Source: CAD feature listing. Evaluate the final solid. Frame: model axes, mm. Coordinates: 2 decimals unless noted, no trailing zeros. Order: outer loops, then holes, each group sorted by start corner. A loop starts at its lowest first (then second) coordinate and runs counter-clockwise, first axis right, second up.
```python
from build123d import *

# Parameters (mm, degrees)
MODEL_R             = 0.65
MODEL_R_2           = 2.974594
EXTRUDE_1_DEPTH     = 1
CUT_EXTRUDE_1_DEPTH = 0.1


with BuildPart() as part:
    # Model → Бобышка-Вытянуть1 (new body)
    with BuildSketch(Plane.XY):
        with BuildLine():
            Line((-10.4, -5.5), (-4.7, -5.5))
            Line((-4.7, -5.5), (-0.65, -5.5))
            Line((-0.65, -5.5), (-0.65, -4.7))
            ThreePointArc((-0.65, -4.7), (0, -4.05), (0.65, -4.7))
            Line((0.65, -4.7), (0.65, -5.5))
            Line((0.65, -5.5), (3.6, -5.5))
            Line((3.6, -5.5), (5.6, -5.5))
            ThreePointArc((5.6, -5.5), (6.660660172, -5.060660172), (7.1, -4))
            Line((7.1, -4), (7.1, -1.6))
            Line((7.1, -1.6), (7.1, 1.6))
            Line((7.1, 1.6), (7.1, 4))
            ThreePointArc((7.1, 4), (6.660660172, 5.060660172), (5.6, 5.5))
            Line((5.6, 5.5), (3.6, 5.5))
            Line((3.6, 5.5), (0.65, 5.5))
            Line((0.65, 5.5), (0.65, 4.7))
            ThreePointArc((0.65, 4.7), (0, 4.05), (-0.65, 4.7))
            Line((-0.65, 4.7), (-0.65, 5.5))
            Line((-0.65, 5.5), (-4.7, 5.5))
            Line((-4.7, 5.5), (-10.4, 5.5))
            ThreePointArc((-10.4, 5.5), (-11.460660172, 5.060660172), (-11.9, 4))
            Line((-11.9, 4), (-11.9, 2.6))
            Line((-11.9, 2.6), (-11.9, 1.5))
            Line((-11.9, 1.5), (-11.9, 1))
            Line((-11.9, 1), (-11.9, -1))
            Line((-11.9, -1), (-11.9, -1.5))
            Line((-11.9, -1.5), (-11.9, -2.6))
            Line((-11.9, -2.6), (-11.9, -4))
            ThreePointArc((-11.9, -4), (-11.460660172, -5.060660172), (-10.4, -5.5))
        make_face()
        with Locations((5.6, -4)):
            Circle(MODEL_R, mode=Mode.SUBTRACT)
        Circle(MODEL_R_2, mode=Mode.SUBTRACT)
        with Locations((5.6, 4)):
            Circle(MODEL_R, mode=Mode.SUBTRACT)
        with Locations((-10.4, -4)):
            Circle(MODEL_R, mode=Mode.SUBTRACT)
        with Locations((-10.4, 4)):
            Circle(MODEL_R, mode=Mode.SUBTRACT)
    extrude(amount=-EXTRUDE_1_DEPTH)

    # Model<3> → Вырез-Вытянуть1 (cut)
    with BuildSketch(Plane.XY):
        Polygon((-11.9, -2.7), (-11.9, -2.900000006), (-9.000000006, -2.900000006), (-9.000000006, -3.800000006), (-4.899999994, -3.800000006), (-4.899999994, 3.800000006), (-9.000000006, 3.800000006), (-9.000000006, 2.900000006), (-11.9, 2.900000006), (-11.9, 2.7), (-8.8, 2.7), (-8.8, 3.6), (-5.1, 3.6), (-5.1, 1.35), (-11.9, 1.35), (-11.9, 1.15), (-5.1, 1.15), (-5.1, -1.15), (-11.9, -1.15), (-11.9, -1.35), (-5.1, -1.35), (-5.1, -3.6), (-8.8, -3.6), (-8.8, -2.7), align=None)
        Polygon((3.799999994, -1.900000006), (7.1, -1.900000006), (7.1, -1.7), (4, -1.7), (4, 1.7), (7.1, 1.7), (7.1, 1.900000006), (3.799999994, 1.900000006), align=None)
    extrude(amount=-CUT_EXTRUDE_1_DEPTH, mode=Mode.SUBTRACT)


solid = part.part
```
Q1. Material intervals for line 1 along Y through (x, z) = (5.6, -0.5); line 2 along Y through (x, z) = (0, -0.35); line 3 along X through (y, z) = (-3.75, -0.45), sorted ascending.
Solutions:
line 1: y = -5.5 to -4.65, -3.35 to 3.35, 4.65 to 5.5
line 2: y = -4.05 to -2.97, 2.97 to 4.05
line 3: x = -11.9 to -11, -9.8 to 5, 6.2 to 7.1
Q2. Pull-direction query (Y, two-part tool) for faces 1 (the flat face through (7.1, -0.1, -0.5)), 2 (the cylindrical face through (-10.916, -4.396, -0.493)), 3 (the flat face through (-5.6, -5.5, -0.5)), 4 (the cylindrical face through (-10.916, 3.604, -0.493)); classes: pulls with the +Y half, pulls with the -Y half, needs draft (parallel to the pull), parting line crosses it, or undercut.
Solutions:
face 1: needs draft
face 2: undercut
face 3: pulls with the -Y half
face 4: undercut
Q3. Section query A-A on z = -0.45. Output: boundary loops of the cut face in (x, y).
Solutions:
outline: (-11.9, -4) arc R1.5 ccw to (-10.4, -5.5) - (-0.65, -5.5) - (-0.65, -4.7) arc R0.65 cw to (0.65, -4.7) - (0.65, -5.5) - (5.6, -5.5) arc R1.5 ccw to (7.1, -4) - (7.1, 4) arc R1.5 ccw to (5.6, 5.5) - (0.65, 5.5) - (0.65, 4.7) arc R0.65 cw to (-0.65, 4.7) - (-0.65, 5.5) - (-10.4, 5.5) arc R1.5 ccw to (-11.9, 4) - close; hole circle Ø1.3 at (-10.4, -4); hole circle Ø1.3 at (-10.4, 4); hole circle Ø5.95 at (0, 0); hole circle Ø1.3 at (5.6, -4); hole circle Ø1.3 at (5.6, 4)
Q4. Section query D-D on x = -2. Output: boundary loops of the cut face in (y, z).
Solutions:
outline: (-5.5, -1) - (-2.2, -1) - (-2.2, 0) - (-5.5, 0) - close; (2.2, -1) - (5.5, -1) - (5.5, 0) - (2.2, 0) - close
Q5. Pin query (flat end, axial travel): P1, Ø0.6, axis at y = -5.5, z = -0.5, coming from the -X side; P2, Ø1, axis at x = 5.6, y = 4, coming from the +Z side. Return the tip coordinate at first contact, or that it passes through.
Solutions:
P1: stops at x = -11.3
P2: passes through
Q6. Section query C-C on x = 1.5. Output: boundary loops of the cut face in (y, z), plus the area to 3 significant figures.
Solutions:
outline: (-5.5, -1) - (-2.57, -1) - (-2.57, 0) - (-5.5, 0) - close; (2.57, -1) - (5.5, -1) - (5.5, 0) - (2.57, 0) - close
area: 5.86 mm2
Q7. Section query B-B on y = 0. Output: boundary loops of the cut face in (x, z).
Solutions:
outline: (-11.9, -1) - (-2.97, -1) - (-2.97, 0) - (-4.9, 0) - (-4.9, -0.1) - (-5.1, -0.1) - (-5.1, 0) - (-11.9, 0) - close; (2.97, -1) - (7.1, -1) - (7.1, 0) - (4, 0) - (4, -0.1) - (3.8, -0.1) - (3.8, 0) - (2.97, 0) - close
